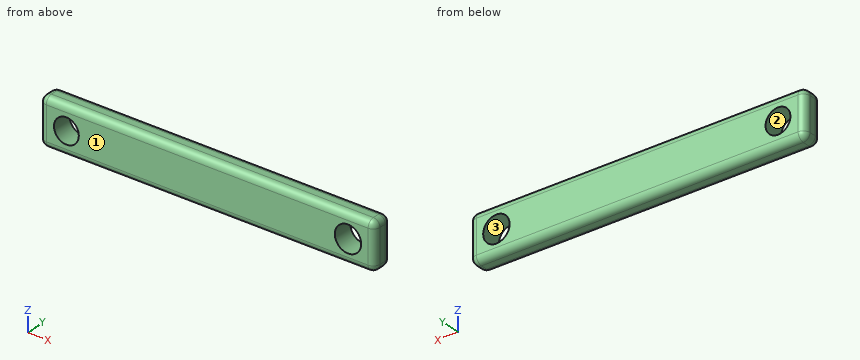
from build123d import *

# Parameters (mm, degrees)
SKETCH1_W           = 63.5
SKETCH1_H           = 8.89
BOSS_EXTRUDE1_DEPTH = 3.81
FILLET1_R           = 1.27
SKETCH2_R           = 2.35
SKETCH2_R_2         = 2.5
CUT_EXTRUDE1_DEPTH  = 41.820799329


with BuildPart() as part:
    # Sketch1 → Boss-Extrude1 (new body)
    with BuildSketch(Plane(origin=(0, 0, 0), x_dir=(1, 0, 0), z_dir=(0, 1, 0))):
        with Locations((-4.799174917, 13.330808581)):
            Rectangle(SKETCH1_W, SKETCH1_H)
    extrude(amount=BOSS_EXTRUDE1_DEPTH)

    # Fillet1
    fillet1_edges = [part.edges().sort_by_distance(p)[0] for p in [
        (26.950825083, 3.81, -13.330808581),
        (-4.799174917, 3.81, -17.775808581),
        (-36.549174917, 3.81, -13.330808581),
        (-4.799174917, 0, -17.775808581),
        (26.950825083, 0, -13.330808581),
        (-4.799174917, 0, -8.885808581),
        (-36.549174917, 0, -13.330808581),
        (-36.549174917, 1.905, -17.775808581),
        (26.950825083, 1.905, -17.775808581),
        (26.950825083, 1.905, -8.885808581),
        (-36.549174917, 1.905, -8.885808581),
        (-4.799174917, 3.81, -8.885808581),
    ]]
    fillet(fillet1_edges, radius=FILLET1_R)

    # Sketch2 → Cut-Extrude1 (cut, through all)
    with BuildSketch(Plane(origin=(0, 3.81, 0), x_dir=(1, 0, 0), z_dir=(0, 1, 0))):
        with Locations(Location((-31.469174917, 13.330808581, 0), (0, 0, 270))):
            Circle(SKETCH2_R)
        with Locations(Location((21.870825083, 13.330808581, 0), (0, 0, 270))):
            Circle(SKETCH2_R_2)
    extrude(amount=-CUT_EXTRUDE1_DEPTH, mode=Mode.SUBTRACT)


solid = part.part
Model file for the job. Use its own axes, mm. Face numbers are marked on the shaded views. Give positions to 0.01 mm unless a question says otherwise; leave off trailing zeros. Order: outer loops, then holes, each group sorted by start corner. A loop starts at its lowest first (then second) coordinate and runs counter-clockwise, first axis right, second up. Notation, with made-up numbers: (17.25, 34) - (33.25, 34) arc R16 ccw to (33.25, 40) - close; hole circle Ø4 at (25.5, -5.75). An arc over 180 degrees is marked (long way). One line per item, written item: value.
Item 1: Slice it at D-D (x = 23). List the corners of the cut face in (y, z).
Response values:
outline: (0, -16.51) arc R1.27 ccw to (1.27, -17.78) - (2.54, -17.78) arc R1.27 ccw to (3.81, -16.51) - (3.81, -15.56) - (0, -15.56) - close; (0, -11.1) - (3.81, -11.1) - (3.81, -10.16) arc R1.27 ccw to (2.54, -8.89) - (1.27, -8.89) arc R1.27 ccw to (0, -10.16) - close
Item 2: Pin check, flat tip, straight feed: pin 1 Ø4 at (x, z) = (21.87, -13.33) entering from +Y. Stop position of the tip, or through.
Response values:
pin 1: through
Item 3: Two-plate mould, pull along X, no slides. Class the marked faces 1, 2 and 3: released by +X, released by -X, zero draft, split by the parting line, or undercut.
Response values:
face 1: zero draft
face 2: undercut
face 3: undercut
Item 4: Slice it at B-B (z = -11.5). List the corners of the cut face in (x, y).
Response values:
outline: (-36.55, 1.27) arc R1.27 ccw to (-35.28, 0) - (-32.94, 0) - (-32.94, 3.81) - (-35.28, 3.81) arc R1.27 ccw to (-36.55, 2.54) - close; (-30, 0) - (20.17, 0) - (20.17, 3.81) - (-30, 3.81) - close; (23.57, 0) - (25.68, 0) arc R1.27 ccw to (26.95, 1.27) - (26.95, 2.54) arc R1.27 ccw to (25.68, 3.81) - (23.57, 3.81) - close
Item 5: Slice it at C-C (y = 3.2). List the corners of the cut face in (x, z).
Response values:
outline: (-36.36, -16.51) arc R1.09 ccw to (-35.28, -17.59) - (25.68, -17.59) arc R1.09 ccw to (26.77, -16.51) - (26.77, -10.16) arc R1.09 ccw to (25.68, -9.07) - (-35.28, -9.07) arc R1.09 ccw to (-36.36, -10.16) - close; hole circle Ø4.7 at (-31.47, -13.33); hole circle Ø5 at (21.87, -13.33)
Item 6: Wall check: line 1 (X direction, y = 1.4, z = -13.5); line 2 (X direction, y = 1.6, z = -13); line 3 (Z direction, x = 20, y = 1.7). Give the ranges that are in metal, low to high.
Response values:
line 1: -36.55 to -33.81, -29.13 to 19.38, 24.37 to 26.95
line 2: -36.55 to -33.8, -29.14 to 19.39, 24.35 to 26.95
line 3: -17.78 to -14.99, -11.67 to -8.89
Item 7: Slice it at A-A (x = -2.5). List the corners of the cut face in (y, z).
Response values:
outline: (0, -16.51) arc R1.27 ccw to (1.27, -17.78) - (2.54, -17.78) arc R1.27 ccw to (3.81, -16.51) - (3.81, -10.16) arc R1.27 ccw to (2.54, -8.89) - (1.27, -8.89) arc R1.27 ccw to (0, -10.16) - close
